CAD build for the part. Positions are in the model's coordinates, mm. Face numbers are marked on the shaded views. A direction names the side the tool comes from. Give positions to 0.01 mm unless a question says otherwise; leave off trailing zeros. Write each loop counter-clockwise with the first axis right and the second up, starting at its lowest first coordinate (ties: lowest second). Pieces come first, ordered by that corner, then holes. Notation, with made-up numbers: (2.5, 64.5) - (36.5, 64.5) arc R30 cw to (36.5, 90.5) - close; hole circle Ø1 at (-2.5, 59). An arc over 180 degrees is marked (long way). Answer as a JSON object with one key per item and string values.
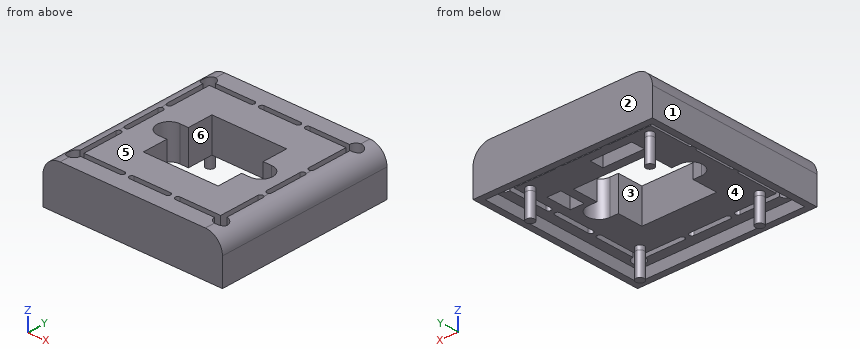
from build123d import *

# Parameters (mm, degrees)
F0_W        = 39
F0_H        = 39
F0_R        = 0.975
F1_DEPTH    = 9
F2_T1_DEPTH = 62
F3_DEPTH    = 5.5
F4_DEPTH    = 1.5
F5_DEPTH    = 2.5
F6_DEPTH    = 1.5
F7_DEPTH    = 5
F8_DEPTH    = 1


# Not quite as in the source:
# - a fillet or chamfer that OpenCascade refuses, or shapes differently, is made with other operations: its cross-section is extruded or revolved along the edge and cut away or added


with BuildPart() as f1:
    # F0 (on Top) → F1 (new body)
    with BuildSketch(Plane.XY):
        Polygon((-2.625, 21), (-21, 21), (-21, -21), (-2.625, -21), (2.625, -21), (21, -21), (21, 21), (2.625, 21), align=None)
        Rectangle(F0_W, F0_H, mode=Mode.SUBTRACT)
        Rectangle(F0_W, F0_H)
        with BuildLine():
            ThreePointArc((16, 4.25), (16.6, 4.85), (17.2, 4.25))
            Line((17.2, 4.25), (17.2, -4.25))
            ThreePointArc((17.2, -4.25), (16.6, -4.85), (16, -4.25))
            Line((16, -4.25), (16, -6.5))
            ThreePointArc((16, -6.5), (16.6, -5.9), (17.2, -6.5))
            Line((17.2, -6.5), (17.2, -15.7))
            ThreePointArc((17.2, -15.7), (18.2606601718, -18.2606601718), (15.7, -17.2))
            Line((15.7, -17.2), (6.5, -17.2))
            ThreePointArc((6.5, -17.2), (5.9, -16.6), (6.5, -16))
            Line((6.5, -16), (4.25, -16))
            ThreePointArc((4.25, -16), (4.85, -16.6), (4.25, -17.2))
            Line((4.25, -17.2), (-4.25, -17.2))
            ThreePointArc((-4.25, -17.2), (-4.85, -16.6), (-4.25, -16))
            Line((-4.25, -16), (-6.5, -16))
            ThreePointArc((-6.5, -16), (-5.9, -16.6), (-6.5, -17.2))
            Line((-6.5, -17.2), (-15.7, -17.2))
            ThreePointArc((-15.7, -17.2), (-18.2606601718, -18.2606601718), (-17.2, -15.7))
            Line((-17.2, -15.7), (-17.2, -6.5))
            ThreePointArc((-17.2, -6.5), (-16.6, -5.9), (-16, -6.5))
            Line((-16, -6.5), (-16, -4.25))
            ThreePointArc((-16, -4.25), (-16.6, -4.85), (-17.2, -4.25))
            Line((-17.2, -4.25), (-17.2, 4.25))
            ThreePointArc((-17.2, 4.25), (-16.6, 4.85), (-16, 4.25))
            Line((-16, 4.25), (-16, 6.5))
            ThreePointArc((-16, 6.5), (-16.6, 5.9), (-17.2, 6.5))
            Line((-17.2, 6.5), (-17.2, 15.7))
            ThreePointArc((-17.2, 15.7), (-18.2606601718, 18.2606601718), (-15.7, 17.2))
            Line((-15.7, 17.2), (-6.5, 17.2))
            ThreePointArc((-6.5, 17.2), (-5.9, 16.6), (-6.5, 16))
            Line((-6.5, 16), (-4.25, 16))
            ThreePointArc((-4.25, 16), (-4.85, 16.6), (-4.25, 17.2))
            Line((-4.25, 17.2), (4.25, 17.2))
            ThreePointArc((4.25, 17.2), (4.85, 16.6), (4.25, 16))
            Line((4.25, 16), (6.5, 16))
            ThreePointArc((6.5, 16), (5.9, 16.6), (6.5, 17.2))
            Line((6.5, 17.2), (15.7, 17.2))
            ThreePointArc((15.7, 17.2), (18.2606601718, 18.2606601718), (17.2, 15.7))
            Line((17.2, 15.7), (17.2, 6.5))
            ThreePointArc((17.2, 6.5), (16.6, 5.9), (16, 6.5))
            Line((16, 6.5), (16, 4.25))
        make_face(mode=Mode.SUBTRACT)
        Polygon((16, -4.25), (16, 4.25), (16, 6.5), (16, 16), (6.5, 16), (4.25, 16), (-4.25, 16), (-6.5, 16), (-16, 16), (-16, 6.5), (-16, 4.25), (-16, -4.25), (-16, -6.5), (-16, -16), (-6.5, -16), (-4.25, -16), (4.25, -16), (6.5, -16), (16, -16), (16, -6.5), align=None)
        with Locations((-14, -14)):
            Circle(F0_R, mode=Mode.SUBTRACT)
        with Locations((14, -14)):
            Circle(F0_R, mode=Mode.SUBTRACT)
        with Locations((-14, 14)):
            Circle(F0_R, mode=Mode.SUBTRACT)
        Polygon((-8.75, 14), (0, 14), (0, 10.75), (-8.75, 10.75), (-9.75, 10.75), (-9.75, 14), align=None, mode=Mode.SUBTRACT)
        with BuildLine():
            Line((-8.75, 8.75), (8.75, 8.75))
            Line((8.75, 8.75), (8.75, 2.75))
            Line((8.75, 2.75), (10.75, 2.75))
            ThreePointArc((10.75, 2.75), (13.5, 0), (10.75, -2.75))
            Line((10.75, -2.75), (8.75, -2.75))
            Line((8.75, -2.75), (8.75, -8.75))
            Line((8.75, -8.75), (-8.75, -8.75))
            Line((-8.75, -8.75), (-8.75, -2.75))
            Line((-8.75, -2.75), (-10.75, -2.75))
            ThreePointArc((-10.75, -2.75), (-13.5, 0), (-10.75, 2.75))
            Line((-10.75, 2.75), (-8.75, 2.75))
            Line((-8.75, 2.75), (-8.75, 8.75))
        make_face(mode=Mode.SUBTRACT)
        Polygon((10.75, 3.8126846775), (10.75, 8.75), (10.75, 9.75), (14, 9.75), (14, 8.75), (14, 3.8126846775), align=None, mode=Mode.SUBTRACT)
        with Locations((14, 14)):
            Circle(F0_R, mode=Mode.SUBTRACT)
        Polygon((0, 10.75), (0, 14), (-8.75, 14), (-9.75, 14), (-9.75, 10.75), (-8.75, 10.75), align=None)
        Polygon((10.75, 9.75), (10.75, 8.75), (10.75, 3.8126846775), (14, 3.8126846775), (14, 8.75), (14, 9.75), align=None)
        with Locations((14, -14)):
            Circle(F0_R)
        with Locations((-14, -14)):
            Circle(F0_R)
        with Locations((-14, 14)):
            Circle(F0_R)
        with Locations((14, 14)):
            Circle(F0_R)
    extrude(amount=F1_DEPTH)

    # F2: fillet of radius 4 on 2 edges, made by hand

    # F2_s2 → F2_t1 (cut)
    with BuildSketch(Plane.XZ.offset(-31)):
        with BuildLine():
            ThreePointArc((-21, 5), (-19.8284271247, 7.8284271247), (-17, 9))
            Line((-17, 9), (-21, 9))
            Line((-21, 9), (-21, 5))
        make_face()
        with BuildLine():
            ThreePointArc((21, 5), (19.8284271247, 7.8284271247), (17, 9))
            Line((17, 9), (21, 9))
            Line((21, 9), (21, 5))
        make_face()
    extrude(amount=F2_T1_DEPTH, mode=Mode.SUBTRACT)

    # F0 (on Top) → F3 (join)
    with BuildSketch(Plane.XY):
        with Locations((-14, -14)):
            Circle(F0_R)
        with Locations((14, -14)):
            Circle(F0_R)
        with Locations((-14, 14)):
            Circle(F0_R)
        with Locations((14, 14)):
            Circle(F0_R)
    extrude(amount=-F3_DEPTH)

    # F0 (on Top) → F4 (join)
    with BuildSketch(Plane.XY):
        Rectangle(F0_W, F0_H)
        with BuildLine():
            ThreePointArc((16, 4.25), (16.6, 4.85), (17.2, 4.25))
            Line((17.2, 4.25), (17.2, -4.25))
            ThreePointArc((17.2, -4.25), (16.6, -4.85), (16, -4.25))
            Line((16, -4.25), (16, -6.5))
            ThreePointArc((16, -6.5), (16.6, -5.9), (17.2, -6.5))
            Line((17.2, -6.5), (17.2, -15.7))
            ThreePointArc((17.2, -15.7), (18.2606601718, -18.2606601718), (15.7, -17.2))
            Line((15.7, -17.2), (6.5, -17.2))
            ThreePointArc((6.5, -17.2), (5.9, -16.6), (6.5, -16))
            Line((6.5, -16), (4.25, -16))
            ThreePointArc((4.25, -16), (4.85, -16.6), (4.25, -17.2))
            Line((4.25, -17.2), (-4.25, -17.2))
            ThreePointArc((-4.25, -17.2), (-4.85, -16.6), (-4.25, -16))
            Line((-4.25, -16), (-6.5, -16))
            ThreePointArc((-6.5, -16), (-5.9, -16.6), (-6.5, -17.2))
            Line((-6.5, -17.2), (-15.7, -17.2))
            ThreePointArc((-15.7, -17.2), (-18.2606601718, -18.2606601718), (-17.2, -15.7))
            Line((-17.2, -15.7), (-17.2, -6.5))
            ThreePointArc((-17.2, -6.5), (-16.6, -5.9), (-16, -6.5))
            Line((-16, -6.5), (-16, -4.25))
            ThreePointArc((-16, -4.25), (-16.6, -4.85), (-17.2, -4.25))
            Line((-17.2, -4.25), (-17.2, 4.25))
            ThreePointArc((-17.2, 4.25), (-16.6, 4.85), (-16, 4.25))
            Line((-16, 4.25), (-16, 6.5))
            ThreePointArc((-16, 6.5), (-16.6, 5.9), (-17.2, 6.5))
            Line((-17.2, 6.5), (-17.2, 15.7))
            ThreePointArc((-17.2, 15.7), (-18.2606601718, 18.2606601718), (-15.7, 17.2))
            Line((-15.7, 17.2), (-6.5, 17.2))
            ThreePointArc((-6.5, 17.2), (-5.9, 16.6), (-6.5, 16))
            Line((-6.5, 16), (-4.25, 16))
            ThreePointArc((-4.25, 16), (-4.85, 16.6), (-4.25, 17.2))
            Line((-4.25, 17.2), (4.25, 17.2))
            ThreePointArc((4.25, 17.2), (4.85, 16.6), (4.25, 16))
            Line((4.25, 16), (6.5, 16))
            ThreePointArc((6.5, 16), (5.9, 16.6), (6.5, 17.2))
            Line((6.5, 17.2), (15.7, 17.2))
            ThreePointArc((15.7, 17.2), (18.2606601718, 18.2606601718), (17.2, 15.7))
            Line((17.2, 15.7), (17.2, 6.5))
            ThreePointArc((17.2, 6.5), (16.6, 5.9), (16, 6.5))
            Line((16, 6.5), (16, 4.25))
        make_face(mode=Mode.SUBTRACT)
    extrude(amount=-F4_DEPTH)

    # F5 (cut): a face of the model
    f5_faces = [f1.faces().sort_by_distance(p)[0] for p in [
        (-18.9484567107, 0, -1.5),
    ]]
    extrude(f5_faces, amount=-F5_DEPTH, mode=Mode.SUBTRACT)

    # F0 (on Top) → F6 (join)
    with BuildSketch(Plane.XY):
        Polygon((-2.625, 21), (-21, 21), (-21, -21), (-2.625, -21), (2.625, -21), (21, -21), (21, 21), (2.625, 21), align=None)
        Rectangle(F0_W, F0_H, mode=Mode.SUBTRACT)
    extrude(amount=-F6_DEPTH)

    # F0 (on Top) → F7 (cut)
    with BuildSketch(Plane.XY):
        Polygon((10.75, 9.75), (10.75, 8.75), (10.75, 3.8126846775), (14, 3.8126846775), (14, 8.75), (14, 9.75), align=None)
        Polygon((0, 10.75), (0, 14), (-8.75, 14), (-9.75, 14), (-9.75, 10.75), (-8.75, 10.75), align=None)
    extrude(amount=F7_DEPTH, mode=Mode.SUBTRACT)

    # F0 (on Top) → F8 (cut)
    with BuildSketch(Plane.XY):
        Polygon((16, -4.25), (16, 4.25), (16, 6.5), (16, 16), (6.5, 16), (4.25, 16), (-4.25, 16), (-6.5, 16), (-16, 16), (-16, 6.5), (-16, 4.25), (-16, -4.25), (-16, -6.5), (-16, -16), (-6.5, -16), (-4.25, -16), (4.25, -16), (6.5, -16), (16, -16), (16, -6.5), align=None)
        with Locations((-14, -14)):
            Circle(F0_R, mode=Mode.SUBTRACT)
        with Locations((14, -14)):
            Circle(F0_R, mode=Mode.SUBTRACT)
        with Locations((-14, 14)):
            Circle(F0_R, mode=Mode.SUBTRACT)
        Polygon((-8.75, 14), (0, 14), (0, 10.75), (-8.75, 10.75), (-9.75, 10.75), (-9.75, 14), align=None, mode=Mode.SUBTRACT)
        with BuildLine():
            Line((-8.75, 8.75), (8.75, 8.75))
            Line((8.75, 8.75), (8.75, 2.75))
            Line((8.75, 2.75), (10.75, 2.75))
            ThreePointArc((10.75, 2.75), (13.5, 0), (10.75, -2.75))
            Line((10.75, -2.75), (8.75, -2.75))
            Line((8.75, -2.75), (8.75, -8.75))
            Line((8.75, -8.75), (-8.75, -8.75))
            Line((-8.75, -8.75), (-8.75, -2.75))
            Line((-8.75, -2.75), (-10.75, -2.75))
            ThreePointArc((-10.75, -2.75), (-13.5, 0), (-10.75, 2.75))
            Line((-10.75, 2.75), (-8.75, 2.75))
            Line((-8.75, 2.75), (-8.75, 8.75))
        make_face(mode=Mode.SUBTRACT)
        Polygon((10.75, 3.8126846775), (10.75, 8.75), (10.75, 9.75), (14, 9.75), (14, 8.75), (14, 3.8126846775), align=None, mode=Mode.SUBTRACT)
        with Locations((14, 14)):
            Circle(F0_R, mode=Mode.SUBTRACT)
    extrude(amount=F8_DEPTH, mode=Mode.SUBTRACT)


solid = f1.part
(1) Pull direction X, two halves, no side cores. Call the marked faces 1, 2 and 3: pulls with the +X half, pulls with the -X half, needs draft (parallel to the pull), parting line crosses it, or undercut.
Answer key:
{"face 1": "pulls with the -X half", "face 2": "needs draft", "face 3": "undercut"}
(2) 3-axis set-ups, long thin cutter, end or side, ignore diameter. For the marked faces 4, 5 and 6: which of +Z, -Z, +X, -X, +Y, -Y reach the whole face in a straight line?
Answer key:
{"face 4": "-Z", "face 5": "+Z, +X, -X, +Y, -Y", "face 6": "+Z, -Z"}
(3) Saw through at C-C, the plane y = 8. Give the cut face in (x, z) (3 decimals).
Answer key:
{"outline": "(-21, -1.5) - (-19.5, -1.5) - (-19.5, 1) - (-17.2, 1) - (-17.2, 8.995) arc R4 ccw to (-21, 5) - close; (-16, 1) - (-8.75, 1) - (-8.75, 9) - (-16, 9) - close; (8.75, 1) - (10.75, 1) - (10.75, 5) - (14, 5) - (14, 1) - (16, 1) - (16, 9) - (8.75, 9) - close; (17.2, 1) - (19.5, 1) - (19.5, -1.5) - (21, -1.5) - (21, 5) arc R4 ccw to (17.2, 8.995) - close"}
(4) Saw through at A-A, the plane z = 0.5. Give the cut face in (x, y) (3 decimals).
Answer key:
{"outline": "(-21, -21) - (21, -21) - (21, 21) - (-21, 21) - close; circle Ø1.95 at (-14, -14); circle Ø1.95 at (-14, 14); circle Ø1.95 at (14, -14); circle Ø1.95 at (14, 14); hole (-19.5, -19.5) - (19.5, -19.5) - (19.5, 19.5) - (-19.5, 19.5) - close"}
(5) Saw through at B-B, the plane x = -14. Give the cut face in (y, z) (3 decimals), and give its area (3 significant figures).
Answer key:
{"outline": "(-21, -1.5) - (-19.5, -1.5) - (-19.5, 1) - (-17.2, 1) - (-17.2, 9) - (-21, 9) - close; (-16, 1) - (-14.975, 1) - (-14.975, -5.5) - (-13.025, -5.5) - (-13.025, 1) - (13.025, 1) - (13.025, -5.5) - (14.975, -5.5) - (14.975, 1) - (16, 1) - (16, 9) - (-16, 9) - close; (17.2, 1) - (19.5, 1) - (19.5, -1.5) - (21, -1.5) - (21, 9) - (17.2, 9) - close", "area": "350 mm²"}
(6) Saw through at D-D, the plane x = 8. Give the cut face in (y, z).
Answer key:
{"outline": "(-21, -1.5) - (-19.5, -1.5) - (-19.5, 1) - (-17.2, 1) - (-17.2, 9) - (-21, 9) - close; (-16, 1) - (-8.75, 1) - (-8.75, 9) - (-16, 9) - close; (8.75, 1) - (16, 1) - (16, 9) - (8.75, 9) - close; (17.2, 1) - (19.5, 1) - (19.5, -1.5) - (21, -1.5) - (21, 9) - (17.2, 9) - close"}
(7) Flat gauge pin, fed straight in: P1, Ø1.5, axis at x = 2.5, y = -9.5, coming from the -Z side. Where does the tip first touch, or does it go through?
Answer key:
{"P1": "stops at z = 1"}
(8) Probe L1, parallel to Y at x = -7, z = 2.5; L2, parallel to Y at x = -8, z = 8; L3, parallel to X at y = 14.5, z = 3. List the from-to ranges inside material, lowest first. Write a range as [from, to].
Answer key:
{"L1": "y = [-21, -17.2], [-16, -8.75], [8.75, 10.75], [14, 16], [17.2, 21]", "L2": "y = [-21, -17.2], [-16, -8.75], [8.75, 16], [17.2, 21]", "L3": "x = [-21, -17.2], [-16, 16], [17.2, 21]"}
